from build123d import *

# Parameters (mm, degrees)
SKETCH1_W                       = 203.2
SKETCH1_H                       = 114.3
BOSS_EXTRUDE1_DEPTH             = 2.794
F_1_8_0_125_DIAMETER_HOLE1_D    = 3.175
F_5_32_0_15625_DIAMETER_HOLE1_D = 3.96875
SKETCH4_W                       = 113.5879999
SKETCH4_H                       = 70.38799994
CUT_EXTRUDE1_DEPTH              = 117.603983362
FILLET1_R                       = 1.524
FILLET2_R                       = 6.35
SKETCH7_R                       = 5.969
CUT_EXTRUDE2_DEPTH              = 117.603983362


with BuildPart() as part:
    # Sketch1 → Boss-Extrude1 (new body)
    with BuildSketch(Plane.XY):
        Rectangle(SKETCH1_W, SKETCH1_H)
    extrude(amount=BOSS_EXTRUDE1_DEPTH)

    # 1/8 (0.125) Diameter Hole1 (through all)
    with Locations(Plane.XY.offset(2.794)):
        with Locations((-82.6, -40.07), (-82.6, 37.53), (44.5, -40.07), (44.5, 37.53)):
            Hole(F_1_8_0_125_DIAMETER_HOLE1_D / 2)

    # 5/32 (0.15625) Diameter Hole1 (through all)
    with Locations(Plane.XY.offset(2.794)):
        with Locations((95.25, -17.78), (-95.25, 50.8), (95.25, 50.8), (95.25, -50.8), (-95.25, -50.8), (-95.25, -17.78)):
            Hole(F_5_32_0_15625_DIAMETER_HOLE1_D / 2)

    # Sketch4 → Cut-Extrude1 (cut, through all)
    with BuildSketch(Plane.XY.offset(2.794)):
        with Locations((-17.78, 1.89000003)):
            Rectangle(SKETCH4_W, SKETCH4_H)
    extrude(amount=-CUT_EXTRUDE1_DEPTH, mode=Mode.SUBTRACT)

    # Fillet1
    fillet1_edges = [part.edges().sort_by_distance(p)[0] for p in [
        (39.01399995, 37.084, 1.397),
        (39.01399995, -33.30399994, 1.397),
        (-74.57399995, -33.30399994, 1.397),
        (-74.57399995, 37.084, 1.397),
    ]]
    fillet(fillet1_edges, radius=FILLET1_R)

    # Fillet2
    fillet2_edges = [part.edges().sort_by_distance(p)[0] for p in [
        (101.6, -57.15, 1.397),
        (-101.6, -57.15, 1.397),
        (-101.6, 57.15, 1.397),
        (101.6, 57.15, 1.397),
    ]]
    fillet(fillet2_edges, radius=FILLET2_R)

    # Sketch7 → Cut-Extrude2 (cut, through all)
    with BuildSketch(Plane.XY.offset(2.794)):
        with Locations((69.85, 19.05)):
            Circle(SKETCH7_R)
        with BuildLine():
            Line((64.135, -21.817900829), (64.135, -16.282099171))
            ThreePointArc((64.135, -16.282099171), (69.85, -12.7), (75.565, -16.282099171))
            Line((75.565, -16.282099171), (75.565, -21.817900829))
            ThreePointArc((75.565, -21.817900829), (69.85, -25.4), (64.135, -21.817900829))
        make_face()
    extrude(amount=-CUT_EXTRUDE2_DEPTH, mode=Mode.SUBTRACT)


solid = part.part
The listing builds one solid part. Answer for the finished solid, in the listing's coordinates (mm). A direction names the side the tool comes from. Give positions to 0.01 mm unless a question says otherwise; leave off trailing zeros. Loops run counter-clockwise (first coordinate to the right, second up) from the corner with the lowest first, then second, coordinate; pieces in that order, holes last. Notation, with made-up numbers: (48.25, -12) - (62.25, -12) arc R26 cw to (62.25, 21) - close; hole circle Ø11 at (-26, -18). An arc over 180 degrees is marked (long way). Answer as a JSON object with one key per item and string values.
1. A cutting plane is placed at A-A (x = 69.85). Write down the section's boundary in (y, z), then the cut area to 3 significant figures.
Determined:
{"outline": "(-57.15, 0) - (-25.4, 0) - (-25.4, 2.79) - (-57.15, 2.79) - close; (-12.7, 0) - (13.08, 0) - (13.08, 2.79) - (-12.7, 2.79) - close; (25.02, 0) - (57.15, 0) - (57.15, 2.79) - (25.02, 2.79) - close", "area": "251 mm²"}
2. A flat-ended cylindrical pin translates along its axis: pin 1 Ø4 at (x, y) = (44.5, 37.53) entering from +Z. Find the tip coordinate at first contact, or state that the pin passes through.
Determined:
{"pin 1": "z = 2.79"}
3. Find the intervals of material crossed by L1, parallel to Y at x = -95.25, z = 1.8; L2, parallel to Y at x = -82.6, z = 1.55; L3, parallel to Y at x = -47, z = 0.5, in increasing order. Write a range as [from, to].
Determined:
{"L1": "[-57.15, -52.78], [-48.82, -19.76], [-15.8, 48.82], [52.78, 57.15]", "L2": "[-57.15, -41.66], [-38.48, 35.94], [39.12, 57.15]", "L3": "[-57.15, -33.3], [37.08, 57.15]"}
4. A cutting plane is placed at B-B (z = 2.15). Give the number of separate pieces and of enclosed holes in the cut face, then the cut area to 3 significant figures.
Determined:
{"separate pieces": "1", "enclosed holes": "13", "area": "14,900 mm²"}
5. For a pull along Y with two mould halves and no side action, classify faces 1 (the cylindrical face through (75.364, 16.764, 1.417)), 2 (the cylindrical face through (-97.1, -18.5, 1.4)), 3 (the cylindrical face through (99.69, -55.34, 1.42)), 4 (the flat face through (44, 1, 2.794)) as pulls with the +Y half, pulls with the -Y half, needs draft (parallel to the pull), parting line crosses it, or undercut.
Determined:
{"face 1": "undercut", "face 2": "undercut", "face 3": "pulls with the -Y half", "face 4": "needs draft"}
6. A cutting plane is placed at C-C (y = 6.5). Write down the section's boundary in (x, z), then the cut area to 3 significant figures.
Determined:
{"outline": "(-101.6, 0) - (-74.57, 0) - (-74.57, 2.79) - (-101.6, 2.79) - close; (39.01, 0) - (101.6, 0) - (101.6, 2.79) - (39.01, 2.79) - close", "area": "250 mm²"}
7. For faces 5 (the cylindrical face through (-99.79, 55.24, 1.42)), 6 (the cylindrical face through (69.9, -25.4, 1.4)), determine the directions among +Z, -Z, +X, -X, +Y, -Y from which every point of the face is accessible in a straight line to the end or side of a thin tool.
Determined:
{"face 5": "+Z, -Z, -X, +Y", "face 6": "+Z, -Z"}
8. A cutting plane is placed at D-D (x = -16). Write down the section's boundary in (y, z).
Determined:
{"outline": "(-57.15, 0) - (-33.3, 0) - (-33.3, 2.79) - (-57.15, 2.79) - close; (37.08, 0) - (57.15, 0) - (57.15, 2.79) - (37.08, 2.79) - close"}
